```python
from build123d import *

# Parameters (mm, degrees)
SKETCH1_R           = 20
BOSS_EXTRUDE1_DEPTH = 150
SKETCH2_R           = 4
BOSS_EXTRUDE2_DEPTH = 30
BOSS_EXTRUDE3_START = -210
SKETCH3_R           = 4
BOSS_EXTRUDE3_DEPTH = 25


with BuildPart() as part:
    # Sketch1 → Boss-Extrude1 (new body)
    with BuildSketch(Plane(origin=(0, 0, 0), x_dir=(1, 0, 0), z_dir=(0, 1, 0))):
        with Locations(Location((0, 0, 0), (0, 0, 270))):
            Circle(SKETCH1_R)
    extrude(amount=BOSS_EXTRUDE1_DEPTH)

    # Sketch2 → Boss-Extrude2 (add)
    with BuildSketch(Plane.XZ):
        with Locations(Location((0, 0, 0), (0, 0, 90))):
            Circle(SKETCH2_R)
    boss_extrude2 = extrude(amount=BOSS_EXTRUDE2_DEPTH)

    # Mirror1: Boss-Extrude2 across plane
    add(boss_extrude2.mirror(Plane(origin=(0, 75, 0), x_dir=(0, 0, 1), z_dir=(0, -1, 0))))

    # Sketch3 → Boss-Extrude3 (add)
    with BuildSketch(Plane.XZ.offset(30).offset(BOSS_EXTRUDE3_START)):
        with Locations(Location((0, 0, 0), (0, 0, 90))):
            Circle(SKETCH3_R)
    extrude(amount=-BOSS_EXTRUDE3_DEPTH)


solid = part.part
```
The listing builds one solid part. Answer for the finished solid, in the listing's coordinates (mm). A direction names the side the tool comes from. Coordinates: 2 decimals unless noted, no trailing zeros. Order: outer loops, then holes, each group sorted by start corner. A loop starts at its lowest first (then second) coordinate and runs counter-clockwise, first axis right, second up. Notation, with made-up numbers: M 33,22 L 73,22 A24 cw 73,36 Z; hole C -32.75,51 d10. An arc over 180 degrees is marked long. Answer as a JSON object with one key per item and string values. Group by question number.
1. Section D-D on x = 12 is taken. Write down the section's boundary in (y, z).
2. Section B-B on z = 0 is taken. Write down the section's boundary in (x, y), then the cut area to 3 significant figures.
3. Section C-C on y = 27 is taken. Write down the section's boundary in (x, z).
4. Straight lines are drawn through the part: line 1 (Y direction, x = -6, z = -1.5); line 2 (X direction, y = 157.5, z = 0.5); line 3 (Z direction, x = 1, y = 45). For each, find the intervals that lie inside material, in ascending order.
5. Section A-A on x = 0 is taken. Write down the section's boundary in (y, z), then the cut area to 3 significant figures.
6. Flat-ended cylindrical pins translate along their axes: P1, Ø12, axis at x = -8, z = 8, coming from the -Y side; P2, Ø1.5, axis at x = -7.5, y = 115.5, coming from the -Z side; P3, Ø12, axis at x = -13, y = 39, coming from the -Z side (3 decimals). Find the tip coordinate at first contact, or state that the pin passes through.
7. A tool of negligible diameter and unlimited length cuts with its end or side. For faces 1 (the flat face through (0, 205, 0)), 2 (the cylindrical face through (3.905, 177.115, -0.867)), 3 (the cylindrical face through (3.905, -14.79, -0.867)), from which of +Z, -Z, +X, -X, +Y, -Y can it reach the whole face along a straight path? Write none if from no direction.
Values follow:
{
 "1": {"outline": "M 0,-16 L 150,-16 L 150,16 L 0,16 Z"},
 "2": {"outline": "M -20,0 L -4,0 L -4,-30 L 4,-30 L 4,0 L 20,0 L 20,150 L 4,150 L 4,205 L -4,205 L -4,150 L -20,150 Z", "area": "6,680 mm2"},
 "3": {"outline": "C 0,0 d40"},
 "4": {"line 1": "0 to 150", "line 2": "-3.97 to 3.97", "line 3": "-19.97 to 19.97"},
 "5": {"outline": "M -30,-4 L 0,-4 L 0,-20 L 150,-20 L 150,-4 L 205,-4 L 205,4 L 150,4 L 150,20 L 0,20 L 0,4 L -30,4 Z", "area": "6,680 mm2"},
 "6": {"P1": "y = 0", "P2": "z = -18.83", "P3": "z = -18.735"},
 "7": {"face 1": "+Z, -Z, +X, -X, +Y", "face 2": "+Y", "face 3": "-Y"}
}
